The model under review builds one solid part; all positions refer to its coordinate system, in mm. Face numbers are marked on the shaded views. A direction names the side the tool comes from. Coordinates: 2 decimals unless noted, no trailing zeros. Write each loop counter-clockwise with the first axis right and the second up, starting at its lowest first coordinate (ties: lowest second). Pieces come first, ordered by that corner, then holes. Notation, with made-up numbers: (76.5, -16.75) -> (91.5, -16.75) arc R6 cw to (91.5, -9.75) -> close; hole circle Ø3 at (35, 62). An arc over 180 degrees is marked (long way). Write each question's results on one line, items separated by ' | '.
```python
from build123d import *

# Parameters (mm, degrees)
SKETCH001_R          = 52
SKETCH001_R_2        = 2
PAD001_DEPTH         = 3
SKETCH_R             = 27
SKETCH_R_2           = 24
PAD_DEPTH            = 12
SKETCH002_R          = 1.8
POCKET_DEPTH         = 5
BODY_PLACEMENT_ANGLE = 180


with BuildPart() as part:
    # Sketch001 → Pad001 (new body)
    with BuildSketch(Plane.XY):
        Circle(SKETCH001_R)
        Circle(SKETCH001_R_2, mode=Mode.SUBTRACT)
    extrude(amount=-PAD001_DEPTH)

    # Sketch → Pad (join)
    with BuildSketch(Plane.XY):
        Circle(SKETCH_R)
        Circle(SKETCH_R_2, mode=Mode.SUBTRACT)
    extrude(amount=PAD_DEPTH)

    # Sketch002 → Pocket (cut)
    with BuildSketch(Plane.XY):
        with Locations((5.656854, 5.656854)):
            Circle(SKETCH002_R)
        with Locations((-5.656854, 5.656854)):
            Circle(SKETCH002_R)
        with Locations((-5.656854, -5.656854)):
            Circle(SKETCH002_R)
        with Locations((5.656854, -5.656854)):
            Circle(SKETCH002_R)
    extrude(amount=-POCKET_DEPTH, mode=Mode.SUBTRACT)


with BuildPart() as part_1:
    # Body placement: moved
    add(part.part.moved(Location((0, 0, 63))).rotate(Axis((0, 0, 63), (0, 0, -1)), BODY_PLACEMENT_ANGLE))


solid = part_1.part
```
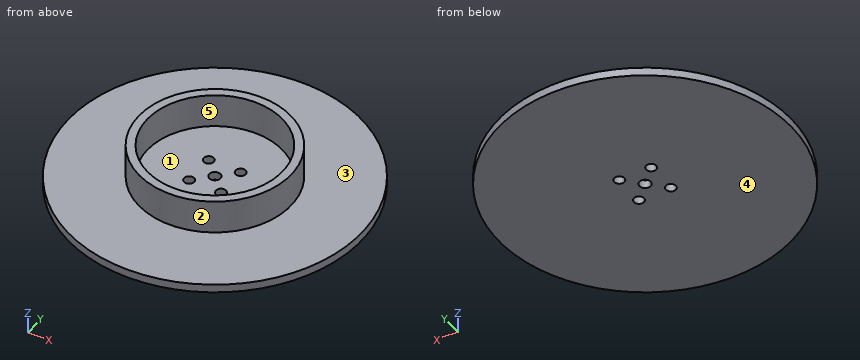
Q1. Add section D-D (y = -16). Write out the cut boundary in (x, z).
Solution:
outline: (-49.48, 60) -> (49.48, 60) -> (49.48, 63) -> (21.75, 63) -> (21.75, 75) -> (17.89, 75) -> (17.89, 63) -> (-17.89, 63) -> (-17.89, 75) -> (-21.75, 75) -> (-21.75, 63) -> (-49.48, 63) -> close
Q2. Add section C-C (z = 73). Write out the cut boundary in (x, y).
Solution:
outline: circle Ø54 at (0, 0); hole circle Ø48 at (0, 0)
Q3. Add section A-A (x = 0). Write out the cut boundary in (y, z), plus the area to 3 significant figures.
Solution:
outline: (-52, 60) -> (-2, 60) -> (-2, 63) -> (-24, 63) -> (-24, 75) -> (-27, 75) -> (-27, 63) -> (-52, 63) -> close; (2, 60) -> (52, 60) -> (52, 63) -> (27, 63) -> (27, 75) -> (24, 75) -> (24, 63) -> (2, 63) -> close | area: 372 mm²
Q4. Machinability: for the marked faces 4 and 5, which of the approach directions +Z, -Z, +X, -X, +Y, -Y give a long, thin tool a straight path to every point of the face, cutting with its end or side? Answer none if there is none.
Solution:
face 4: -Z, +X, -X, +Y, -Y | face 5: +Z
Q5. Clearance check with flat-ended pins moving along their axes: P1, Ø6, axis at x = 5.66, y = -5.66, coming from the +Z side; P2, Ø1.5, axis at y = -23.5, z = 71.5, coming from the -X side; P3, Ø8, axis at x = -1.5, z = 68, coming from the +Y side. State where each tip first meets the part, or that it passes through.
Solution:
P1: z = 63 | P2: x = -14.54 | P3: y = 27
Q6. Draft analysis for pull direction Y (two halves, no side actions). For the marked faces 1, 2 and 3, state which applies: pulls with the +Y half, pulls with the -Y half, needs draft (parallel to the pull), parting line crosses it, or undercut.
Solution:
face 1: undercut | face 2: parting line crosses it | face 3: needs draft
Q7. For line 1 (X direction, y = 0, z = 61.7); line 2 (Y direction, x = -1, z = 70.25), list the stretches that pass through material, from the lowest coordinate up. Write a range as from..to.
Solution:
line 1: -52..-2, 2..52 | line 2: -26.98..-23.98, 23.98..26.98
